CAD build for the part. Positions are in the model's coordinates, mm. A direction names the side the tool comes from. Round coordinates to 2 decimals unless told otherwise and drop trailing zeros. Order: outer loops, then holes, each group sorted by start corner. A loop starts at its lowest first (then second) coordinate and runs counter-clockwise, first axis right, second up.
```python
from build123d import *

# Parameters (mm, degrees)
F_3_8_NPT_TAPPED_HOLE1_AT_2_COUNT = 2
F_3_8_NPT_TAPPED_HOLE1_AT_2_PITCH = 76.2
F_3_8_CLEARANCE_HOLE2_D           = 10.0838
CIRPATTERN1_COUNT                 = 10
SKETCH15_R                        = 3.175
CUT_EXTRUDE1_DEPTH                = 12.7
SKETCH18_R                        = 1.27
CUT_EXTRUDE2_DEPTH                = 3.302


with BuildPart() as part:
    # Sketch1 → Revolve1 (revolve)
    with BuildSketch(Plane.XY):
        Polygon((0, 0), (-76.2, 0), (-76.2, -38.1), (-60.96, -38.1), (-60.96, -32.258), (-55.7149, -32.258), (-55.7149, -29.5656), (-51.6509, -29.5656), (-51.6509, -32.258), (-32.163982831, -32.258), (-30.364664072, -32.258), (-28.575, -32.258), (-28.575, -27.178), (-28.0924, -27.178), (-28.0924, -24.4856), (-24.0284, -24.4856), (-24.0284, -27.178), (-22.225, -27.178), (0, -15.85722), align=None)
    revolve(axis=Axis((0, 0, 0), (0, -1, 0)))

    # Sketch3 → 1/2 NPT Tapped Hole1 (revolve, cut)
    with BuildSketch(Plane(origin=(0, 0, 0), x_dir=(0, 0, 1), z_dir=(1, 0, 0))):
        Polygon((0, 0), (0, 38.1), (8.9281, 38.1), (8.9281, 13.462), (10.261665792, 13.462), (10.6647361, 0), align=None)
    revolve(axis=Axis((0, 6.35, 0), (0, -1, 0)), mode=Mode.SUBTRACT)

    # Sketch5 → 3/8 NPT Tapped Hole1 (revolve, cut)
    with BuildSketch(Plane(origin=(-38.1, 0, 0), x_dir=(0, 0, 1), z_dir=(1, 0, 0))):
        Polygon((0, 0), (0, 38.1), (7.1374, 38.1), (7.1374, 10.414), (8.263205494, 10.414), (8.5750146, 0), align=None)
    f_3_8_npt_tapped_hole1 = revolve(axis=Axis((-38.1, 6.35, 0), (0, -1, 0)), mode=Mode.SUBTRACT)

    # 3/8 NPT Tapped Hole1 at 2: 3/8 NPT Tapped Hole1 ×2
    with Locations(*[(i * F_3_8_NPT_TAPPED_HOLE1_AT_2_PITCH, 0, 0) for i in range(1, F_3_8_NPT_TAPPED_HOLE1_AT_2_COUNT)]):
        add(f_3_8_npt_tapped_hole1, mode=Mode.SUBTRACT)

    # 3/8 Clearance Hole2 (through all)
    with Locations(Plane(origin=(67.31, 0, 0), x_dir=(1, 0, 0), z_dir=(0, 1, 0))):
        with Locations((0, 0)):
            f_3_8_clearance_hole2 = Hole(F_3_8_CLEARANCE_HOLE2_D / 2)

    # CirPattern1: 3/8 Clearance Hole2 ×10 about axis
    cirpattern1_axis = Axis((0, 0, 0), (0, 1, 0))
    for i in range(1, CIRPATTERN1_COUNT):
        add(f_3_8_clearance_hole2.rotate(cirpattern1_axis, i * 360 / CIRPATTERN1_COUNT), mode=Mode.SUBTRACT)

    # Sketch7 → 1/8 NPT Tapped Hole2 (revolve, cut)
    with BuildSketch(Plane(origin=(19.05, 0, -33.02), x_dir=(0, 0, 1), z_dir=(1, 0, 0))):
        Polygon((0, 0), (0, 38.1), (4.2164, 38.1), (4.2164, 6.858), (4.556413846, 6.858), (4.7427388, 0.635), (5.3777388, 0), align=None)
    revolve(axis=Axis((19.05, 6.35, -33.02), (0, -1, 0)), mode=Mode.SUBTRACT)

    # Sketch15 → Cut-Extrude1 (cut, symmetric)
    with BuildSketch(Plane(origin=(0, -4.272551224, -4.272551224), x_dir=(0, 0.7071067811865489, -0.7071067811865461), z_dir=(0, -0.7071067811865461, -0.7071067811865489))):
        with Locations((-30.172299887, 0)):
            Circle(SKETCH15_R)
    extrude(amount=CUT_EXTRUDE1_DEPTH, both=True, mode=Mode.SUBTRACT)

    # Sketch12 → 1/8 NPT Tapped Hole3 (revolve, cut)
    with BuildSketch(Plane(origin=(0, 0, 26.67), x_dir=(0, 0, 1), z_dir=(1, 0, 0))):
        Polygon((0, 0), (0, 20.32), (4.2164, 17.786531286), (4.2164, 6.858), (4.543696598, 6.858), (4.7427388, 0.2102612), (4.953, 0), align=None)
    revolve(axis=Axis((0, 6.35, 26.67), (0, -1, 0)), mode=Mode.SUBTRACT)

    # Sketch17 → 1/4 NPT Tapped Hole1 (revolve, cut)
    with BuildSketch(Plane(origin=(-19.05, 0, -33.02), x_dir=(0, 0, 1), z_dir=(1, 0, 0))):
        Polygon((0, 0), (0, 38.1), (5.5626, 38.1), (5.5626, 9.906), (5.962698545, 9.906), (6.2402847, 0.635), (6.8752847, 0), align=None)
    revolve(axis=Axis((-19.05, 6.35, -33.02), (0, -1, 0)), mode=Mode.SUBTRACT)

    # Sketch18 → Cut-Extrude2 (cut)
    with BuildSketch(Plane.XZ.offset(32.258)):
        with Locations((0, 44.45)):
            Circle(SKETCH18_R)
        with Locations((0, -44.45)):
            Circle(SKETCH18_R)
    extrude(amount=-CUT_EXTRUDE2_DEPTH, mode=Mode.SUBTRACT)


solid = part.part
```
1. Pin check, flat tips, straight feed: P1, Ø6, axis at y = -28.5, z = -42.5, coming from the -X side; P2, Ø1.5, axis at y = -26, z = 45, coming from the +X side; P3, Ø5, axis at x = -4, y = -20.5, coming from the -Z side. Stop position of each tip, or through.
2. Cut at C-C, the plane z = 48.5. Write the cut outline in (x, y), and give its area (3 significant figures).
3. Mould opens along Z. For faces 1 (the face through (71.31, -19.32, 3.07)), 2 (the face through (-2.682, -16.885, 8.516)), 3 (the face through (57, -38.1, -23)) say: released by +Z, released by -Z, zero draft, split by the parting line, or undercut.
4. Cut at B-B, the plane x = -67.31. Write the cut outline in (y, z), and give its area (3 significant figures).
5. Cut at A-A, the plane z = 0. Give the number of separate pieces and of enclosed holes in the cut face, and give its area (3 significant figures).
6. Drill centre lines: line 1 (X direction, y = -9, z = 5.5); line 2 (X direction, y = -16, z = -33); line 3 (Z direction, x = 19, y = -13). Where is each one in solid material? Low to high.
7. Tool access for faces 4 (the face through (-13.62, -20.93, -34.23)), 5 (the face through (5.209, -25.851, 23.457)), 6 (the face through (41, -10.414, 7)): list every direction of +Z, -Z, +X, -X, +Y, -Y with a clear straight run to the whole face (end or side of a thin tool).
Outcome:
1. P1: stops at x = -65.16
1. P2: stops at x = 62.04
1. P3: stops at z = -76.19
2. outline: (-58.77, -38.1) - (-36.93, -38.1) - (-36.93, -32.26) - (-27.42, -32.26) - (-27.42, -29.57) - (-17.76, -29.57) - (-17.76, -32.26) - (17.76, -32.26) - (17.76, -29.57) - (27.42, -29.57) - (27.42, -32.26) - (36.93, -32.26) - (36.93, -38.1) - (58.77, -38.1) - (58.77, 0) - (-58.77, 0) - close
2. area: 3,990 mm2
3. face 1: undercut
3. face 2: undercut
3. face 3: zero draft
4. outline: (-38.1, -35.72) - (0, -35.72) - (0, -5.04) - (-38.1, -5.04) - close; (-38.1, 5.04) - (0, 5.04) - (0, 35.72) - (-38.1, 35.72) - close
4. area: 2,340 mm2
5. separate pieces: 6
5. enclosed holes: 0
5. area: 2,400 mm2
6. line 1: x = -76 to -44.32, -31.88 to -8.82, 8.82 to 31.88, 44.32 to 76
6. line 2: x = -68.68 to -24.61, -13.49 to 14.83, 23.27 to 68.68
6. line 3: z = -73.79 to -68.73, -59.31 to -37.24, -28.8 to 59.31, 68.73 to 73.79
7. face 4: +Y, -Y
7. face 5: -Y
7. face 6: +Y
